```python
from build123d import *

# Parameters (mm, degrees)
SKETCH_1_R               = 48.25
EXTRUDE_1_DEPTH          = 30
CUT_EXTRUDE_1_DEPTH      = 75.539419102
CUT_EXTRUDE_1_DEPTH_BACK = 75.539419102
CUT_EXTRUDE_2_DEPTH      = 75.539419102
CUT_EXTRUDE_2_DEPTH_BACK = 75.539419102
CUT_EXTRUDE_3_DEPTH      = 75.539419102
CUT_EXTRUDE_3_DEPTH_BACK = 75.539419102
SKETCH_3_R               = 1.9
CUT_EXTRUDE_START        = 5
SKETCH_4_OUTSIDE_W       = 116.544
SKETCH_4_OUTSIDE_H       = 125.27
SKETCH_4_OUTSIDE_R       = 38.5
CUT_EXTRUDE_4_DEPTH      = 20
RIB_4_REACH              = 76.539
SKETCH_8_WALL_W          = 171.078838204
SKETCH_8_WALL_H          = 5
PATTERN_CIRCULAR_1_COUNT = 5
PATTERN_CIRCULAR_1_ANGLE = 180


with BuildPart() as part:
    # Sketch 1 → Extrude 1 (new body)
    with BuildSketch(Plane.XY):
        Circle(SKETCH_1_R)
    extrude(amount=EXTRUDE_1_DEPTH)

    # Sketch 2 → Cut-Extrude 1 (cut, two sides: drawn at the far end of the back side and taken through both)
    with BuildSketch(Plane.XY.offset(30).offset(-CUT_EXTRUDE_1_DEPTH_BACK)):
        with BuildLine():
            Line((28.67032155, -20.075175272), (0, 0))
            Line((0, 0), (6.077686218, 34.468271355))
            ThreePointArc((6.077686218, 34.468271355), (-32.335783638, -13.393920133), (28.67032155, -20.075175272))
        make_face()
    extrude(amount=CUT_EXTRUDE_1_DEPTH + CUT_EXTRUDE_1_DEPTH_BACK, mode=Mode.SUBTRACT)

    # Sketch 2_3 → Cut-Extrude 2 (cut, two sides: drawn at the far end of the back side and taken through both)
    with BuildSketch(Plane.XY.offset(30).offset(-CUT_EXTRUDE_2_DEPTH_BACK)):
        Polygon((50.420697892, 285.949987287), (8.378524572, 47.516974083), (0, 0), (39.524086137, -27.675063054), (237.849992482, -166.544357699), (685.21320647, 18.759552842), (497.78391188, 471.253897827), align=None)
    extrude(amount=CUT_EXTRUDE_2_DEPTH + CUT_EXTRUDE_2_DEPTH_BACK, mode=Mode.SUBTRACT)

    # Sketch 3 → Cut-Extrude 3 (cut, two sides: drawn at the far end of the back side and taken through both)
    with BuildSketch(Plane.XY.offset(-CUT_EXTRUDE_3_DEPTH_BACK)):
        with Locations((31.466251763, 31.466251763)):
            Circle(SKETCH_3_R)
        with Locations((44.5, 0)):
            Circle(SKETCH_3_R)
        with Locations((31.466251763, -31.466251763)):
            Circle(SKETCH_3_R)
        with Locations((-31.466251763, -31.466251763)):
            Circle(SKETCH_3_R)
        with Locations((0, 42.5)):
            Circle(SKETCH_3_R)
        with Locations((0, -42.5)):
            Circle(SKETCH_3_R)
        with Locations((-44.5, 0)):
            Circle(SKETCH_3_R)
        with Locations((-31.466251763, 31.466251763)):
            Circle(SKETCH_3_R)
    extrude(amount=CUT_EXTRUDE_3_DEPTH + CUT_EXTRUDE_3_DEPTH_BACK, mode=Mode.SUBTRACT)

    # Sketch 4 outside → Cut-Extrude 4 (cut)
    with BuildSketch(Plane.XY.offset(CUT_EXTRUDE_START)):
        with Locations((-4.363, 0)):
            Rectangle(SKETCH_4_OUTSIDE_W, SKETCH_4_OUTSIDE_H)
        Circle(SKETCH_4_OUTSIDE_R, mode=Mode.SUBTRACT)
    extrude(amount=CUT_EXTRUDE_4_DEPTH, mode=Mode.SUBTRACT)

    # Sketch 8 wall → Rib 4 (add, up to next)
    with BuildSketch(Plane(origin=(17.794779605, -42.960398262, 15), x_dir=(0, 0, 1), z_dir=(0.382683432365, -0.923879532511, 0)), mode=Mode.PRIVATE) as rib_4_sk1:
        Rectangle(SKETCH_8_WALL_W, SKETCH_8_WALL_H)
    rib_4_tool1 = extrude(rib_4_sk1.sketch, amount=-RIB_4_REACH, mode=Mode.PRIVATE) - part.part
    rib_4 = rib_4_tool1.solids().sort_by_distance((17.794779605, -42.960398262, 15))[0]
    add(rib_4)

    # Pattern Circular 1: Rib 4 ×5 about axis
    pattern_circular_1_axis = Axis((0, 0, 0), (0, 0, -1))
    for i in range(1, PATTERN_CIRCULAR_1_COUNT):
        add(rib_4.rotate(pattern_circular_1_axis, i * PATTERN_CIRCULAR_1_ANGLE / (PATTERN_CIRCULAR_1_COUNT - 1)))


solid = part.part
```
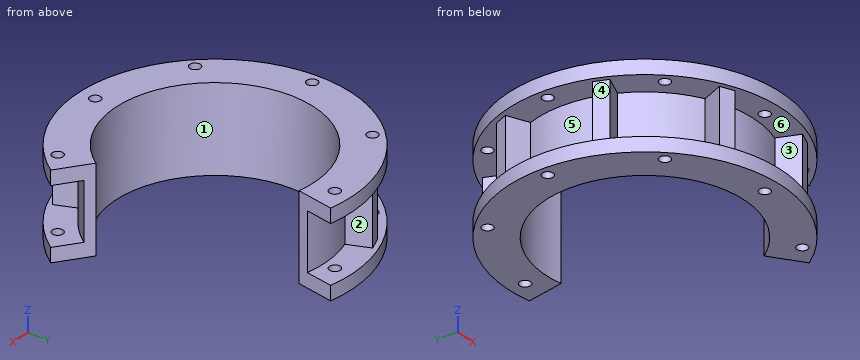
Read the model definition and answer for the solid it produces. Units are mm, in the model's axes. Face numbers are marked on the shaded views. A direction names the side the tool comes from. Coordinates: 2 decimals unless noted, no trailing zeros. Write each loop counter-clockwise with the first axis right and the second up, starting at its lowest first coordinate (ties: lowest second). Pieces come first, ordered by that corner, then holes. Notation, with made-up numbers: (43.25, 41.5) - (57.25, 41.5) arc R27 cw to (57.25, 65.5) - close; hole circle Ø8 at (-37, -20.75). An arc over 180 degrees is marked (long way). Answer as a JSON object with one key per item and string values. Group by question number.
1. A cutting plane is placed at A-A (y = 0). Determine the outline of the cut face in (x, z).
2. A cutting plane is placed at B-B (x = 0). Give the number of separate pieces and of enclosed holes in the cut face, plus the area to 3 significant figures.
3. A cutting plane is placed at C-C (y = -19). Determine the outline of the cut face in (x, z).
4. A cutting plane is placed at D-D (z = 9). Determine the outline of the cut face in (x, y).
5. The mould has two halves that part along Y. Classify the marked faces 1, 2 and 3: +Y half, -Y half, draft (parallel to the pull), parting line (faces both ways), or undercut.
6. Each of these flat-tipped pins is pushed along its axis until it touches: P1, Ø2.5, axis at x = -44.5, y = 0, coming from the +Z side; P2, Ø1, axis at y = 33, z = 6.5, coming from the -X side; P3, Ø4, axis at y = -22, z = 13.5, coming from the -X side; P4, Ø6, axis at x = 6.5, z = 8.5, coming from the +Y side. Where does it stop, or does it pass through?
7. Consider L1, parallel to Y at x = 0, z = 2.15; L2, parallel to X at y = 0, z = 27.05; L3, parallel to Y at x = -1, z = 17. Determine where each line is inside the solid, lowest interval first. Write a range as [from, to].
8. Which of the six approach directions +Z, -Z, +X, -X, +Y, -Y give full straight-line access (tool end or side, diameter ignored) to the marked faces 4, 5 and 6?
Worked out:
{
 "1": {"outline": "(-48.25, 0) - (-46.4, 0) - (-46.4, 5) - (-48.25, 5) - close; (-48.25, 25) - (-46.4, 25) - (-46.4, 30) - (-48.25, 30) - close; (-42.6, 0) - (-35, 0) - (-35, 30) - (-42.6, 30) - (-42.6, 25) - (-38.5, 25) - (-38.5, 5) - (-42.6, 5) - close"},
 "2": {"separate pieces": "6", "enclosed holes": "0", "area": "329 mm²"},
 "3": {"outline": "(-44.35, 0) - (-29.39, 0) - (-29.39, 30) - (-44.35, 30) - (-44.35, 25) - (-42.46, 25) - (-42.46, 5) - (-44.35, 5) - close; hole (-39.34, 5) - (-33.49, 5) - (-33.49, 25) - (-39.34, 25) - close"},
 "4": {"outline": "(-43.92, -15.49) - (-42, -20.1) - (-34.54, -17.01) arc R38.5 ccw to (-17.01, -34.54) - (-20.1, -42) - (-15.49, -43.92) - (-12.39, -36.45) arc R38.5 ccw to (12.39, -36.45) - (15.49, -43.92) - (20.1, -42) - (17.01, -34.54) arc R38.5 ccw to (31.54, -22.08) - (28.67, -20.08) arc R35 cw (long way) to (6.08, 34.47) - (6.69, 37.92) arc R38.5 ccw to (-12.39, 36.45) - (-15.49, 43.92) - (-20.1, 42) - (-17.01, 34.54) arc R38.5 ccw to (-34.54, 17.01) - (-42, 20.1) - (-43.92, 15.49) - (-36.45, 12.39) arc R38.5 ccw to (-36.45, -12.39) - close"},
 "5": {"face 1": "undercut", "face 2": "+Y half", "face 3": "-Y half"},
 "6": {"P1": "passes through", "P2": "stops at x = -20.64", "P3": "stops at x = -42.05", "P4": "stops at y = 38.34"},
 "7": {"L1": "y = [-48.25, -44.4], [-40.6, -35], [35, 40.6], [44.4, 48.25]", "L2": "x = [-48.25, -46.4], [-42.6, -35]", "L3": "y = [-38.49, -34.99], [34.99, 38.49]"},
 "8": {"face 4": "-X, -Y", "face 5": "-X", "face 6": "none"}
}
